from build123d import *

# Parameters (mm, degrees)
F0_R     = 40
F0_R_2   = 20
F1_DEPTH = 40
F2_SIZE  = 5
F3_SIZE  = 2


with BuildPart() as f1:
    # F0 (on Top) → F1 (new body)
    with BuildSketch(Plane.XY):
        Circle(F0_R)
        Circle(F0_R_2, mode=Mode.SUBTRACT)
    extrude(amount=F1_DEPTH)

    # F2
    f2_edges = [f1.edges().sort_by_distance(p)[0] for p in [
        (-40, 0, 40),
    ]]
    chamfer(f2_edges, length=F2_SIZE)

    # F3
    f3_edges = [f1.edges().sort_by_distance(p)[0] for p in [
        (-20, 0, 40),
    ]]
    chamfer(f3_edges, length=F3_SIZE)


solid = f1.part
Design review of the part built by this model. Coordinates are the model's own, in mm. Give positions to 0.01 mm unless a question says otherwise; leave off trailing zeros. Order: outer loops, then holes, each group sorted by start corner. A loop starts at its lowest first (then second) coordinate and runs counter-clockwise, first axis right, second up.
1. Add section A-A, the plane y = 0. State the section outline as (x, z) points.
Solution:
outline: (-40, 0) - (-20, 0) - (-20, 38) - (-22, 40) - (-35, 40) - (-40, 35) - close; (20, 0) - (40, 0) - (40, 35) - (35, 40) - (22, 40) - (20, 38) - close
2. Mouldability with a two-part tool opening along Y and no side actions: class faces 1 (the cylindrical face through (-4.336, -19.524, 18.734)), 2 (the cylindrical face through (-8.67, -39.05, 17.26)), 3 (the flat face through (-9.4, 18.3, 0)) as +Y half, -Y half, draft (parallel to the pull), parting line (faces both ways), or undercut.
Solution:
face 1: undercut
face 2: parting line
face 3: draft
3. Add section C-C, the plane z = 21. State the section outline as (x, y) points.
Solution:
outline: circle Ø80 at (0, 0); hole circle Ø40 at (0, 0)
4. To check wall thickness, follow L1, parallel to Y at x = 0, z = 28.5; L2, parallel to Y at x = -15, z = 30; L3, parallel to X at y = -9, z = 21.5. State the ranges of each line that lie inside material, in increasing order.
Solution:
L1: y = -40 to -20, 20 to 40
L2: y = -37.08 to -13.23, 13.23 to 37.08
L3: x = -38.97 to -17.86, 17.86 to 38.97
5. For pin 1 Ø1 at (x, z) = (-23.5, 18) entering from -Y; pin 2 Ø6 at (y, z) = (24.5, 14.5) entering from -X; pin 3 Ø6 at (y, z) = (-26, 30) entering from -X; pin 4 Ø5 at (x, y) = (31.5, -26.5) entering from -Z, all flat-tipped, find the tip position at first contact; note any pin that passes through.
Solution:
pin 1: stops at y = -32.73
pin 2: stops at x = -33.73
pin 3: stops at x = -32.73
pin 4: stops at z = 0
